The listing builds one solid part. Answer for the finished solid, in the listing's coordinates (mm). Round coordinates to 2 decimals unless told otherwise and drop trailing zeros. Return JSON: item names as keys, results as strings. Group by question number.
(1) The part is cut by section A-A (z = 65.5). Count the separate pieces of the cut face and the enclosed holes in it, plus the area to 3 significant figures.
(2) Consider line 1 (X direction, y = -4, z = 502.5); line 2 (Y direction, x = 8.5, z = 523). Determine where each line is inside the solid, lowest interval first. Write a range as [from, to].
(3) Each of these flat-tipped pins is pushed along its axis until it touches: pin 1 (6 mm diameter, centred on y = -0.5, z = 350.5, fed in from -X); pin 2 (1.6 mm diameter, centred on y = 0.5, z = 179.5, fed in from +X); pin 3 (3 mm diameter, centred on x = 2.5, z = 298.5, fed in from +Y). Where does it stop, or does it pass through?
Autodesk Inventor part; units mm, degrees
ref_plane "Начальная плоскость" through (0, 0, 10) normal (0, 0, 1) x (1, 0, 0)
ref_plane "Конечная плоскость" through (0, 0, 590) normal (0, 0, 1) x (1, 0, 0)
ref_plane "РабПлоскость5" through (281.5, 0, 10) normal (0, 0, -1) x (-1, 0, 0)
ref_plane "Начальная плоскость" through (0, 0, 10) normal (0, 0, 1) x (1, 0, 0)
ref_plane "Конечная плоскость" through (0, 0, 590) normal (0, 0, 1) x (1, 0, 0)
sketch "Эскиз" plane through (0, 0, 0) normal (0, 0, 1) x (1, 0, 0)
  line L0 (-14.4349, 0) -> (14.4349, 0)
  line L1 (0, -14) -> (0, 14)
  line L2 (0, 0) -> (7.5, 7.5) construction
  circle A0 centre (7.5, 7.5) radius 1.65 construction
  line L3 (5.85, 9.15) -> (9.15, 9.15)
  line L4 (9.15, 9.15) -> (9.15, 5.85)
  line L5 (9.15, 5.85) -> (5.85, 5.85)
  line L6 (5.85, 5.85) -> (5.85, 9.15)
  line L7 (3.235, 8.1636) -> (4.72, 9.9636)
  line L8 (4.7971, 10) -> (8.5, 10)
  line L9 (3.3121, 8) -> (4.95, 8)
  line L10 (4.95, 8) -> (4.95, 5.7985)
  line L11 (4.95, 5.7985) -> (2.6515, 3.5)
  line L12 (0, 3.5) -> (2.6515, 3.5)
  circle A1 centre (0, 0) radius 2.5
  line L13 (8.1636, 3.235) -> (9.9636, 4.72)
  line L14 (10, 4.7971) -> (10, 8.5)
  line L15 (8, 3.3121) -> (8, 4.95)
  line L16 (8, 4.95) -> (5.7985, 4.95)
  line L17 (5.7985, 4.95) -> (3.5, 2.6515)
  line L18 (3.5, 0) -> (3.5, 2.6515)
  arc A2 (10, 8.5) -> (8.5, 10) centre (8.5, 8.5) ccw
  line L19 (0, 0) -> (-7.5, 7.5) construction
  circle A3 centre (-7.5, 7.5) radius 1.65 construction
  line L20 (-5.85, 9.15) -> (-9.15, 9.15)
  line L21 (-9.15, 9.15) -> (-9.15, 5.85)
  line L22 (-9.15, 5.85) -> (-5.85, 5.85)
  line L23 (-5.85, 5.85) -> (-5.85, 9.15)
  line L24 (-3.235, 8.1636) -> (-4.72, 9.9636)
  line L25 (-4.7971, 10) -> (-8.5, 10)
  line L26 (-3.3121, 8) -> (-4.95, 8)
  line L27 (-4.95, 8) -> (-4.95, 5.7985)
  line L28 (-4.95, 5.7985) -> (-2.6515, 3.5)
  line L29 (0, 3.5) -> (-2.6515, 3.5)
  line L30 (-3.5, 0) -> (-3.5, 2.6515)
  line L31 (-5.7985, 4.95) -> (-3.5, 2.6515)
  line L32 (-8, 4.95) -> (-5.7985, 4.95)
  line L33 (-8, 3.3121) -> (-8, 4.95)
  line L34 (-8.1636, 3.235) -> (-9.9636, 4.72)
  line L35 (-10, 4.7971) -> (-10, 8.5)
  arc A4 (-8.5, 10) -> (-10, 8.5) centre (-8.5, 8.5) ccw
  line L36 (0, 14) -> (0, -14)
  line L37 (0, 0) -> (7.5, -7.5) construction
  circle A5 centre (7.5, -7.5) radius 1.65 construction
  line L38 (5.85, -9.15) -> (9.15, -9.15)
  line L39 (9.15, -9.15) -> (9.15, -5.85)
  line L40 (9.15, -5.85) -> (5.85, -5.85)
  line L41 (5.85, -5.85) -> (5.85, -9.15)
  line L42 (3.235, -8.1636) -> (4.72, -9.9636)
  line L43 (4.7971, -10) -> (8.5, -10)
  line L44 (3.3121, -8) -> (4.95, -8)
  line L45 (4.95, -8) -> (4.95, -5.7985)
  line L46 (4.95, -5.7985) -> (2.6515, -3.5)
  line L47 (0, -3.5) -> (2.6515, -3.5)
  line L48 (3.5, 0) -> (3.5, -2.6515)
  line L49 (5.7985, -4.95) -> (3.5, -2.6515)
  line L50 (8, -4.95) -> (5.7985, -4.95)
  line L51 (8, -3.3121) -> (8, -4.95)
  line L52 (8.1636, -3.235) -> (9.9636, -4.72)
  line L53 (10, -4.7971) -> (10, -8.5)
  arc A6 (8.5, -10) -> (10, -8.5) centre (8.5, -8.5) ccw
  line L54 (0, 0) -> (-7.5, -7.5) construction
  line L55 (-4.95, -8) -> (-4.95, -5.7985)
  line L56 (-3.3121, -8) -> (-4.95, -8)
  line L57 (-5.7985, -4.95) -> (-3.5, -2.6515)
  line L58 (-4.95, -5.7985) -> (-2.6515, -3.5)
  line L59 (-3.5, 0) -> (-3.5, -2.6515)
  line L60 (0, -3.5) -> (-2.6515, -3.5)
  circle A7 centre (-7.5, -7.5) radius 1.65 construction
  line L61 (-5.85, -5.85) -> (-5.85, -9.15)
  line L62 (-5.85, -9.15) -> (-9.15, -9.15)
  line L63 (-9.15, -9.15) -> (-9.15, -5.85)
  line L64 (-9.15, -5.85) -> (-5.85, -5.85)
  line L65 (-3.235, -8.1636) -> (-4.72, -9.9636)
  line L66 (-8, -4.95) -> (-5.7985, -4.95)
  line L67 (-8, -3.3121) -> (-8, -4.95)
  line L68 (-8.1636, -3.235) -> (-9.9636, -4.72)
  line L69 (-4.7971, -10) -> (-8.5, -10)
  line L70 (-10, -4.7971) -> (-10, -8.5)
  arc A8 (-10, -8.5) -> (-8.5, -10) centre (-8.5, -8.5) ccw
  arc A9 (3.235, 8.1636) -> (3.3121, 8) centre (3.3121, 8.1) ccw
  arc A10 (4.7971, 10) -> (4.72, 9.9636) centre (4.7971, 9.9) ccw
  arc A11 (8, 3.3121) -> (8.1636, 3.235) centre (8.1, 3.3121) ccw
  arc A12 (9.9636, 4.72) -> (10, 4.7971) centre (9.9, 4.7971) ccw
  arc A13 (-3.3121, 8) -> (-3.235, 8.1636) centre (-3.3121, 8.1) ccw
  arc A14 (-4.72, 9.9636) -> (-4.7971, 10) centre (-4.7971, 9.9) ccw
  arc A15 (-8.1636, 3.235) -> (-8, 3.3121) centre (-8.1, 3.3121) ccw
  arc A16 (-10, 4.7971) -> (-9.9636, 4.72) centre (-9.9, 4.7971) ccw
  arc A17 (-8, -3.3121) -> (-8.1636, -3.235) centre (-8.1, -3.3121) ccw
  arc A18 (-9.9636, -4.72) -> (-10, -4.7971) centre (-9.9, -4.7971) ccw
  arc A19 (-3.235, -8.1636) -> (-3.3121, -8) centre (-3.3121, -8.1) ccw
  arc A20 (-4.7971, -10) -> (-4.72, -9.9636) centre (-4.7971, -9.9) ccw
  arc A21 (4.72, -9.9636) -> (4.7971, -10) centre (4.7971, -9.9) ccw
  arc A22 (3.3121, -8) -> (3.235, -8.1636) centre (3.3121, -8.1) ccw
  arc A23 (8.1636, -3.235) -> (8, -3.3121) centre (8.1, -3.3121) ccw
  arc A24 (10, -4.7971) -> (9.9636, -4.72) centre (9.9, -4.7971) ccw
  point P0 (3.1, 8)
  point P1 (4.75, 10)
  point P2 (7.5, 9.15)
  point P3 (8, 3.1)
  point P4 (10, 4.75)
  point P5 (7.5, 5.85)
  point P6 (9.15, 7.5)
  point P7 (-3.1, 8)
  point P8 (-4.75, 10)
  point P9 (-7.5, 9.15)
  point P10 (-8, 3.1)
  point P11 (-10, 4.75)
  point P12 (-7.5, 5.85)
  point P13 (-9.15, 7.5)
  point P14 (3.1, -8)
  point P15 (4.75, -10)
  point P16 (7.5, -9.15)
  point P17 (8, -3.1)
  point P18 (10, -4.75)
  point P19 (7.5, -5.85)
  point P20 (9.15, -7.5)
  point P21 (-3.1, -8)
  point P22 (-7.5, -5.85)
  point P23 (-7.5, -9.15)
  point P24 (-9.15, -7.5)
  point P25 (-4.75, -10)
  point P26 (-8, -3.1)
  point P27 (-10, -4.75)
  dimension "d0" = 45
  dimension "d1" = 3.3
  dimension "d2" = 1.5
  dimension "d3" = 1.2
  dimension "d4" = 5
  dimension "d5" = 6.5
  dimension "d6" = 15
  dimension "d7" = 20
  dimension "d8" = 9.9
  dimension "d9" = 9.5
  dimension "d10" = 6.2
  dimension "d11" = 2
  dimension "d18" = 0.1
  dimension "d19" = 0.1
extrude "Тело" add sketch "Эскиз" along normal up to surface (580 mm away) from surface at 10 contours A1 L1 L12 L11 L10 L9 A9 L7 A10 L8 A2 L14 A12 L13 A11 L15 L16 L17 L18 L0 | L0 L48 L49 L50 L51 A23 L52 A24 L53 A6 L43 A21 L42 A22 L44 L45 L46 L47 L1 A1 | A1 L0 L30 L31 L32 L33 A15 L34 A16 L35 A4 L25 A14 L24 A13 L26 L27 L28 L29 L1 | L1 L60 L58 L55 L56 A19 L65 A20 L69 A8 L70 A18 L68 A17 L67 L66 L57 L59 L0 A1
sketch "Эскиз2" plane through (0, 0, 0) normal (0, 0, 1) x (1, 0, 0)
  line L0 (0, 0) -> (10, 0)
ref_plane "РабПлоскость3" through (0, 0, 0) normal (0, -1, 0) x (1, 0, 0)
sketch "Эскиз3" plane through (0, 0, 0) normal (0, -1, 0) x (1, 0, 0)
  line L0 (-2, 10) -> (12, 10)
  line L1 (-2, 590) -> (12, 590)
  dimension "d25" = 580
ref_plane "РабПлоскость5" through (281.5, 0, 10) normal (0, 0, -1) x (-1, 0, 0)
split "Разделение2" plane through (281.5, 0, 10) removes the side toward (0, 0, -1)
ref_plane "РабПлоскость6" through (0, 0, 10) normal (0, 0, -1) x (-1, 0, 0)
split "Разделение3" plane through (0, 0, 10) removes the side toward (0, 0, -1)
ref_plane "РабПлоскость7" through (0, 0, 590) normal (0, 0, 1) x (1, 0, 0)
split "Разделение4" plane through (0, 0, 590) removes the side toward (0, 0, 1)
ref_plane "РабПлоскость8" through (0, 10, 610) normal (0, 0, 1) x (1, 0, 0)
split "Разделение5" plane through (0, 10, 610) removes the side toward (0, 0, 1)
properties part number "короткая палка"
Answer below:
{
 "1": {"separate pieces": "1", "enclosed holes": "5", "area": "115 mm²"},
 "2": {"line 1": "x = [-9.09, -8], [-4.85, -3.15], [3.15, 4.85], [8, 9.09]", "line 2": "y = [-10, -9.15], [-5.85, -3.51], [3.51, 5.85], [9.15, 10]"},
 "3": {"pin 1": "stops at x = -8.48", "pin 2": "stops at x = 3.5", "pin 3": "stops at y = 9.09"}
}
